Geometry: see drawing. Coordinates: mm, zero at the bounding-box minimum. Give positions to 0.01 mm unless a question says otherwise; leave off trailing zeros. Write each loop counter-clockwise with the first axis right and the second up, starting at its lowest first coordinate (ties: lowest second). Pieces come first, ordered by that corner, then holes. Notation, with made-up numbers: M -16.5,18.5 L 12.5,18.5 A21 ccw 12.5,55.5 Z; hole C -28.5,87.5 d5. An arc over 180 degrees is marked long. Use a Markdown table: item, result. Add a question column.
1) Section A-A on y = 0.8. Return the cut outline in (x, z) (1 decimal), then the cut area to 3 significant figures.
2) Draft query along Z for the marked faces 1, 2, 3 and 4. Return one class per face: +Z half, -Z half, draft (parallel to the pull), parting line (faces both ways), or undercut.
3) Line query: line 1 (Z direction, x = 2.5, y = 0.75); line 2 (Z direction, x = 7.5, y = 2.5); line 3 (Z direction, x = 3.5, y = 2.4). Output: solid intervals per line, ascending.
4) Section C-C on z = 18. Return the cut outline in (x, y) (1 decimal), then the cut area to 3 significant figures.
5) Section B-B on x = 12. Return the cut outline in (y, z), then the cut area to 3 significant figures.
6) Pin query (flat end, axial travel): pin 1 (1.5 mm diameter, centred on x = 12.5, y = 1.5, fed in from +Z); pin 2 (1 mm diameter, centred on y = 2, z = 18.5, fed in from -X). Return the tip coordinate at first contact, or that it passes through.
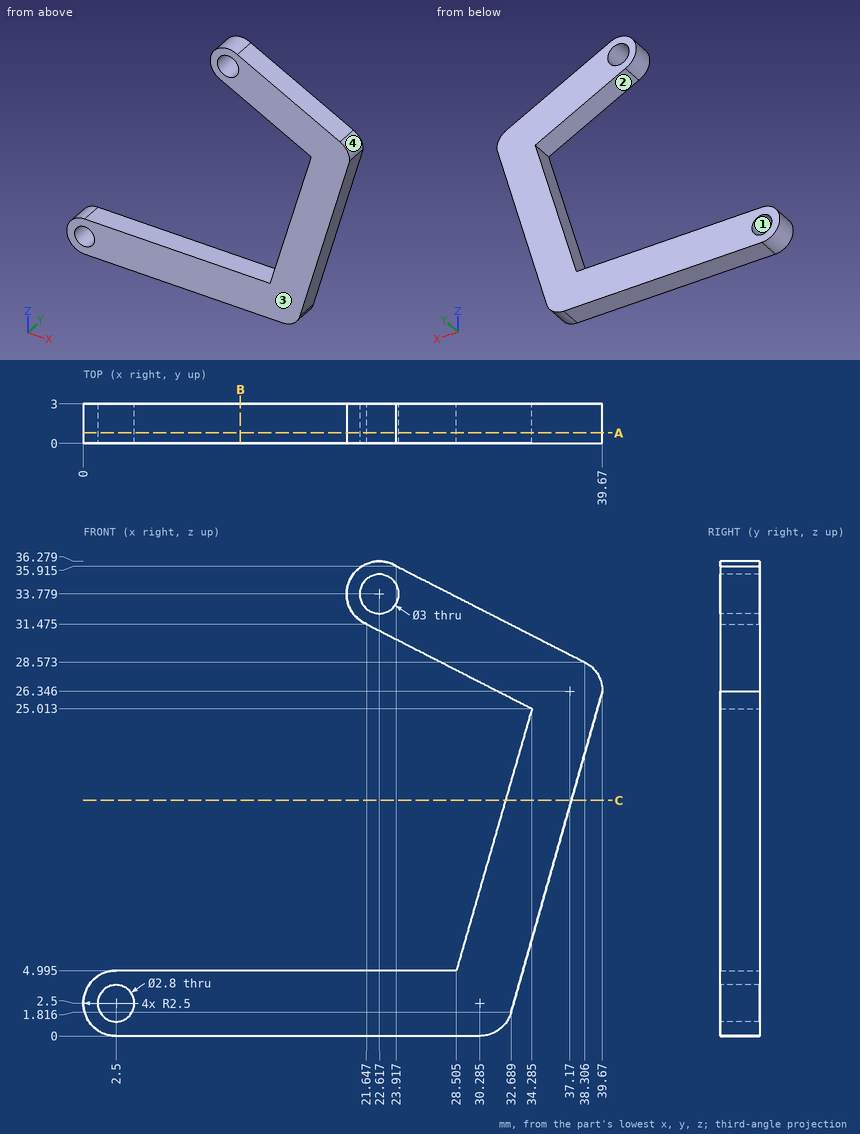
Found:
| question | item | result |
|---|---|---|
| 1 | outline | M 2.5,0 L 30.3,0 A2.5 ccw 32.7,1.8 L 39.7,26.3 A2.5 ccw 38.3,28.6 L 23.9,35.9 A2.5 ccw long 21.6,31.5 L 34.3,25 L 28.5,5 L 2.5,5 A2.5 ccw Z; hole C 2.5,2.5 d2.8; hole C 22.6,33.8 d3 |
| 1 | area | 346 mm² |
| 2 | face 1 | undercut |
| 2 | face 2 | undercut |
| 2 | face 3 | draft |
| 2 | face 4 | +Z half |
| 3 | line 1 | 0 to 1.1, 3.9 to 5 |
| 3 | line 2 | 0 to 5 |
| 3 | line 3 | 0 to 1.52, 3.48 to 5 |
| 4 | outline | M 32.3,0 L 37.3,0 L 37.3,3 L 32.3,3 Z |
| 4 | area | 15.1 mm² |
| 5 | outline | M 0,0 L 3,0 L 3,5 L 0,5 Z |
| 5 | area | 15.0 mm² |
| 6 | pin 1 | z = 5 |
| 6 | pin 2 | x = 32.26 |
